Study the drawing (mm; zero at the part's minimum x, y, z) and answer. A direction names the side the tool comes from. Coordinates: 2 decimals unless noted, no trailing zeros. Order: outer loops, then holes, each group sorted by start corner. A loop starts at its lowest first (then second) coordinate and runs counter-clockwise, first axis right, second up. Notation, with made-up numbers: M -35,28 L 22,28 A19 cw 22,45 Z; hole C 55.25,-37.75 d4. An arc over 180 degrees is marked long. One line per item, written item: value. Start each with the question number.
Q1. The part is cut by section A-A on x = 2.2. Give the vertices of the cut face in (y, z), then the cut area to 3 significant figures.
Q2. For the marked faces 1, 2 and 3, determine the directions among +Z, -Z, +X, -X, +Y, -Y from which every point of the face is accessible in a straight line to the end or side of a thin tool.
Q3. The part is cut by section B-B on z = 2.2. Give the vertices of the cut face in (x, y), then the cut area to 3 significant figures.
Q4. The part is cut by section C-C on y = 7. Give the vertices of the cut face in (x, z), then the cut area to 3 significant figures.
Q5. Straight lines are drawn through the part: line 1 along Y through (x, z) = (1.7, 3.75); line 2 along X through (y, z) = (2.75, 2.7); line 3 along Z through (x, y) = (3.4, 6.75). For each, find the intervals that lie inside material, in ascending order. Write a range as [from, to].
Q6. The part is cut by section D-D on x = 0.35. Give the vertices of the cut face in (y, z).
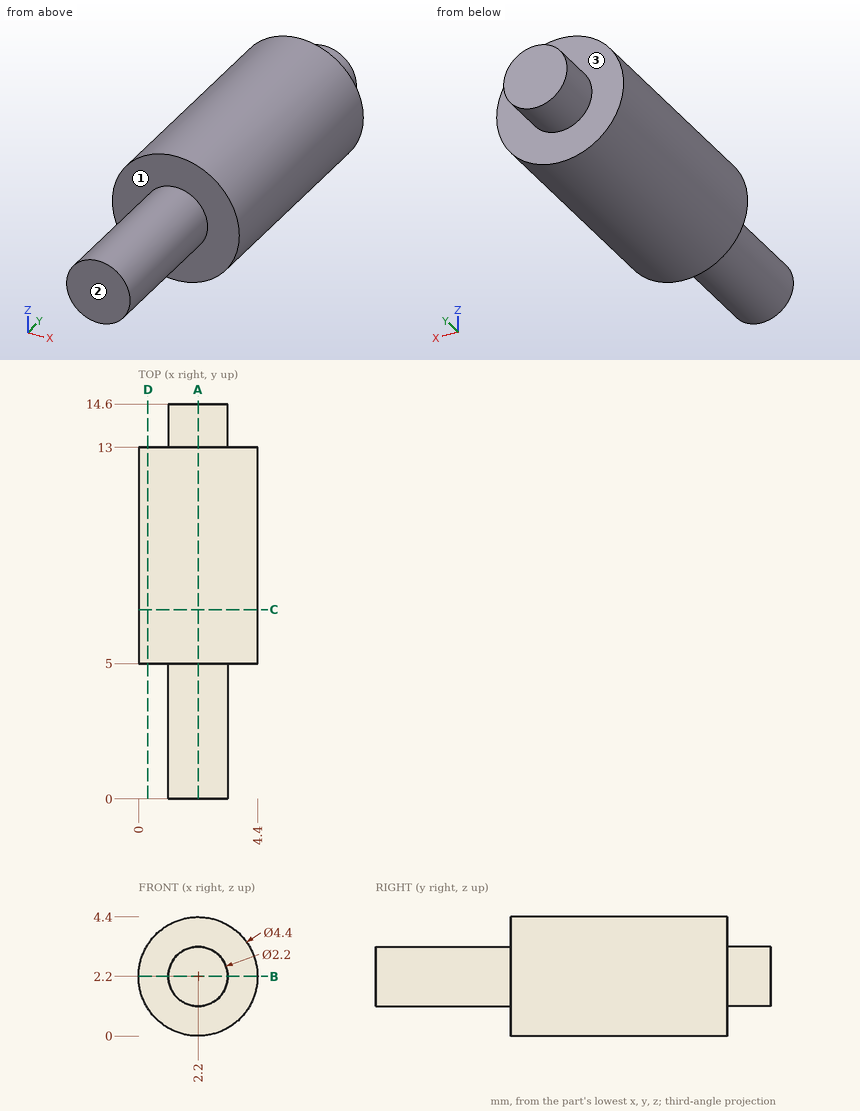
Output:
1. outline: M 0,1.1 L 5,1.1 L 5,0 L 13,0 L 13,1.1 L 14.6,1.1 L 14.6,3.3 L 13,3.3 L 13,4.4 L 5,4.4 L 5,3.3 L 0,3.3 Z
1. area: 49.7 mm^2
2. face 1: -Y
2. face 2: +Z, -Z, +X, -X, -Y
2. face 3: +Y
3. outline: M 0,5 L 1.1,5 L 1.1,0 L 3.3,0 L 3.3,5 L 4.4,5 L 4.4,13 L 3.3,13 L 3.3,14.6 L 1.1,14.6 L 1.1,13 L 0,13 Z
3. area: 49.7 mm^2
4. outline: C 2.2,2.2 d4.4
4. area: 15.2 mm^2
5. line 1: y = [5, 13]
5. line 2: x = [1.22, 3.18]
5. line 3: z = [0.36, 4.04]
6. outline: M 5,1.01 L 13,1.01 L 13,3.39 L 5,3.39 Z
